The model under review builds one solid part; all positions refer to its coordinate system, in mm. Face numbers are marked on the shaded views. A direction names the side the tool comes from. Coordinates: 2 decimals unless noted, no trailing zeros. Loops run counter-clockwise (first coordinate to the right, second up) from the corner with the lowest first, then second, coordinate; pieces in that order, holes last. Notation, with made-up numbers: (65.25, 89) - (115.25, 89) arc R5 cw to (115.25, 94) - close; hole circle Ø1 at (0, 39). An arc over 180 degrees is marked (long way). Answer in a Markdown table with one row per item. Add a question column.
(1) For P1, Ø1, axis at x = -8.5, z = -15.5, coming from the -Y side; P2, Ø4, axis at x = 5, y = 15, coming from the +Z side; P3, Ø12, axis at x = 2.5, z = -45.5, coming from the -Y side, all flat-tipped, find the tip position at first contact; note any pin that passes through.
(2) We need section A-A on y = 0. Write out the cut boundary in (x, z).
(3) We need section D-D on z = -27. Write out the cut boundary in (x, y), plus the area to 3 significant figures.
(4) We need section B-B on z = -80. Write out the cut boundary in (x, y).
(5) We need section C-C on x = 2.25. Write out the cut boundary in (y, z), plus the area to 3 significant figures.
(6) Machinability: for the marked faces 3 and 4, which of the approach directions +Z, -Z, +X, -X, +Y, -Y give a long, thin tool a straight path to every point of the face, cutting with its end or side? Answer none if there is none.
(7) Mouldability with a two-part tool opening along Z and no side actions: class the marked faces 1 and 2 as +Z half, -Z half, draft (parallel to the pull), parting line (faces both ways), or undercut.
(8) For line 1 along Z through (x, y) = (6, -1); line 2 along Z through (x, y) = (1.75, -3); line 3 along Y through (x, z) = (-6, -58), list the stretches that pass through material, from the lowest coordinate up.
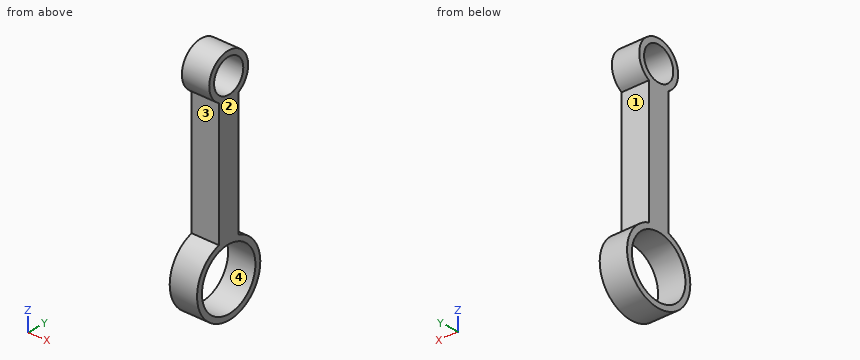
from build123d import *

# Parameters (mm, degrees)
F0_R     = 27.5
F0_R_2   = 15
F1_DEPTH = 12.5


with BuildPart() as f1:
    # F0 (on Right) → F1 (new body, symmetric)
    with BuildSketch(Plane.YZ):
        with BuildLine():
            Line((10, -49.076708), (10, 62.679492))
            ThreePointArc((10, 62.679492), (0, 100), (-10, 62.679492))
            Line((-10, 62.679492), (-10, -49.076708))
            ThreePointArc((-10, -49.076708), (0, -112.5), (10, -49.076708))
        make_face()
        with Locations((0, -80)):
            Circle(F0_R, mode=Mode.SUBTRACT)
        with Locations((0, 80)):
            Circle(F0_R_2, mode=Mode.SUBTRACT)
    extrude(amount=F1_DEPTH, both=True)


solid = f1.part
Outcome:
| question | item | result |
|---|---|---|
| 1 | P1 | y = -10 |
| 1 | P2 | z = 95.2 |
| 1 | P3 | y = -15.62 |
| 2 | outline | (-12.5, -112.5) - (12.5, -112.5) - (12.5, -107.5) - (-12.5, -107.5) - close; (-12.5, -52.5) - (12.5, -52.5) - (12.5, 65) - (-12.5, 65) - close; (-12.5, 95) - (12.5, 95) - (12.5, 100) - (-12.5, 100) - close |
| 3 | outline | (-12.5, -10) - (12.5, -10) - (12.5, 10) - (-12.5, 10) - close |
| 3 | area | 500 mm² |
| 4 | outline | (-12.5, -32.5) - (12.5, -32.5) - (12.5, -27.5) - (-12.5, -27.5) - close; (-12.5, 27.5) - (12.5, 27.5) - (12.5, 32.5) - (-12.5, 32.5) - close |
| 5 | outline | (-10, -49.08) arc R32.5 ccw (long way) to (10, -49.08) - (10, 62.68) arc R20 ccw (long way) to (-10, 62.68) - close; hole circle Ø55 at (0, -80); hole circle Ø30 at (0, 80) |
| 5 | area | 3,670 mm² |
| 6 | face 3 | +X, -X, -Y |
| 6 | face 4 | +X, -X |
| 7 | face 1 | undercut |
| 7 | face 2 | draft |
| 8 | line 1 | -112.48 to -107.48, -52.52 to 65.03, 94.97 to 99.97 |
| 8 | line 2 | -112.36 to -107.34, -52.66 to 65.3, 94.7 to 99.77 |
| 8 | line 3 | -23.92 to -16.5, 16.5 to 23.92 |
